Check sheet for the drawn part. Datum: minimum x, y, z corner. Units: mm. A direction names the side the tool comes from. Give positions to 0.01 mm unless a question says otherwise; leave off trailing zeros. Write each loop counter-clockwise with the first axis right and the second up, starting at its lowest first coordinate (ties: lowest second). Pieces come first, ordered by that corner, then holes. Notation, with made-up numbers: M -4,62 L 23,62 A26 cw 23,95 Z; hole C -24,-6 d9. An arc over 180 degrees is marked long. Write item = value, one per line.
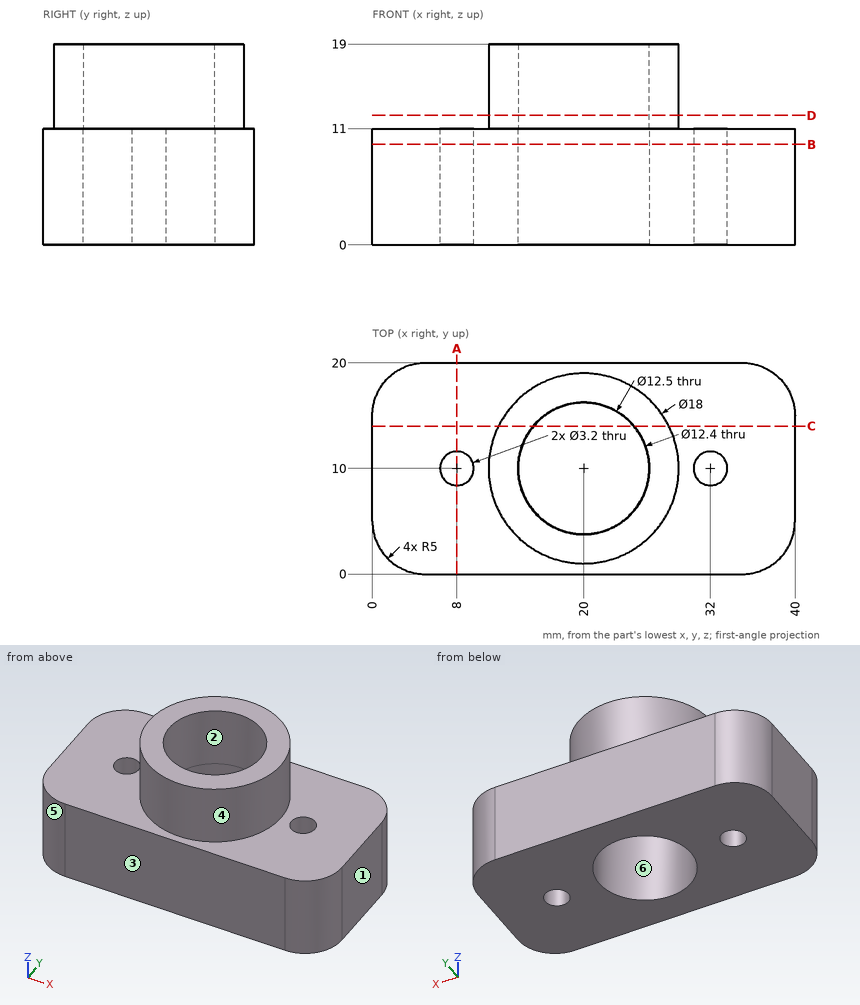
1) Cross-section at B-B on z = 9.5. Record the boundary of the cut face in (x, y).
From the geometry:
outline = M 0,5 A5 ccw 5,0 L 35,0 A5 ccw 40,5 L 40,15 A5 ccw 35,20 L 5,20 A5 ccw 0,15 Z; hole C 8,10 d3.2; hole C 20,10 d12.5; hole C 32,10 d3.2
2) Cross-section at D-D on z = 12.25. Record the boundary of the cut face in (x, y), plus the area to 3 significant figures.
From the geometry:
outline = C 20,10 d18; hole C 20,10 d12.4
area = 134 mm^2
3) Tool access check on the marked faces 4, 5 and 6. Record the directions out of +Z, -Z, +X, -X, +Y, -Y that give a thin tool (end or side, any length) a straight path to the whole face; none if there is none.
From the geometry:
face_4 = +Z
face_5 = +Z, -Z, -X, -Y
face_6 = -Z
4) Draft check along Y on the marked faces 1, 2 and 3. Enter one of: +Y half, -Y half, draft (parallel to the pull), parting line (faces both ways), or undercut.
From the geometry:
face_1 = draft
face_2 = undercut
face_3 = -Y half
5) Cross-section at A-A on x = 8. Record the boundary of the cut face in (y, z), plus the area to 3 significant figures.
From the geometry:
outline = M 0,0 L 8.4,0 L 8.4,11 L 0,11 Z; M 11.6,0 L 20,0 L 20,11 L 11.6,11 Z
area = 185 mm^2
6) Cross-section at C-C on y = 14. Record the boundary of the cut face in (x, z), plus the area to 3 significant figures.
From the geometry:
outline = M 0,0 L 15.2,0 L 15.2,11 L 15.26,11 L 15.26,19 L 11.94,19 L 11.94,11 L 0,11 Z; M 24.74,11 L 24.8,11 L 24.8,0 L 40,0 L 40,11 L 28.06,11 L 28.06,19 L 24.74,19 Z
area = 388 mm^2
7) Material ranges on probe 1 along Y at (x, z) = (32, 5.75); probe 2 along X at (y, z) = (15.25, 8.5); probe 3 along Y at (x, z) = (9, 9), recorded low to high. Write a range as from..to.
From the geometry:
probe_1 = 0..8.4, 11.6..20
probe_2 = 0.01..16.61, 23.39..39.99
probe_3 = 0..8.75, 11.25..20
